```python
from build123d import *

# Parameters (mm, degrees)
F0_R            = 60
F1_DEPTH        = 6
F3_D            = 3.2
F6_D            = 3.2
F6_COPIES_COUNT = 5


# Not quite as in the source:
# - a pattern or mirror of a feature is missing from the dataset's text; its kind, count and spacing are read off the source's solid


with BuildPart() as f1:
    # F0 (on Top) → F1 (new body)
    with BuildSketch(Plane.XY):
        Circle(F0_R)
    extrude(amount=F1_DEPTH)

    # F3 (through all)
    with Locations(Plane.XY.offset(6)):
        with Locations((0, 0)):
            Hole(F3_D / 2)

    # F6 (through all)
    with Locations(Plane.XY.offset(6)):
        with Locations((0, 42.5)):
            f6 = Hole(F6_D / 2)

    # F6_copies: F6 ×5 about axis
    f6_copies_axis = Axis((0, 0, 0), (0, 0, 1))
    for i in range(1, F6_COPIES_COUNT):
        add(f6.rotate(f6_copies_axis, i * 360 / F6_COPIES_COUNT), mode=Mode.SUBTRACT)


solid = f1.part
```
Here's how the part is built. I have some questions about the finished solid (model axes, mm). Give positions to 0.01 mm unless a question says otherwise; leave off trailing zeros. Loops run counter-clockwise (first coordinate to the right, second up) from the corner with the lowest first, then second, coordinate; pieces in that order, holes last. Notation, with made-up numbers: M 76,-16 L 92,-16 A9 ccw 92,-7 Z; hole C 36,-24 d8. An arc over 180 degrees is marked long. Return JSON: item names as keys, results as strings.
Item 1: Imagine slicing it at B-B on x = 0. List the corners of the cut face in (y, z) for me.
A:
{"outline": "M -60,0 L -1.6,0 L -1.6,6 L -60,6 Z; M 1.6,0 L 40.9,0 L 40.9,6 L 1.6,6 Z; M 44.1,0 L 60,0 L 60,6 L 44.1,6 Z"}
Item 2: Please list where these lines run through material, in increasing order: line 1 (Y direction, x = 0, z = 3.6); line 2 (Y direction, x = -1, z = 2.2); line 3 (X direction, y = -33.5, z = 2.5) (3 decimals).
A:
{"line 1": "y = -60 to -1.6, 1.6 to 40.9, 44.1 to 60", "line 2": "y = -59.99 to -1.25, 1.25 to 41.25, 43.75 to 59.99", "line 3": "x = -49.777 to -26.315, -23.647 to 23.647, 26.315 to 49.777"}
Item 3: I'm going to push flat-ended pins straight in: pin 1 Ø2 at (x, z) = (-20, 2.5) entering from -Y; pin 2 Ø1 at (x, z) = (-47.5, 3.5) entering from -Y; pin 3 Ø1.5 at (x, z) = (46, 4.5) entering from -Y. Where does each tip first touch, or does it pass through?
A:
{"pin 1": "stops at y = -56.91", "pin 2": "stops at y = -37.3", "pin 3": "stops at y = -39.4"}
Item 4: Thinking about a two-plate mould opening in Y: for faces 1 (the cylindrical face through (-59.94, 2.64, 2.96)), 2 (the cylindrical face through (41.993, 13.425, 2.958)), 3 (the flat face through (12, 1, 0)), which applies, released by +Y, released by -Y, zero draft, split by the parting line, or undercut?
A:
{"face 1": "split by the parting line", "face 2": "undercut", "face 3": "zero draft"}
Item 5: Imagine slicing it at D-D on y = 42.5. List the corners of the cut face in (x, z) for me, then the cut area to 3 significant figures.
A:
{"outline": "M -42.35,0 L -1.6,0 L -1.6,6 L -42.35,6 Z; M 1.6,0 L 42.35,0 L 42.35,6 L 1.6,6 Z", "area": "489 mm^2"}
Item 6: Imagine slicing it at C-C on z = 2.65. List the corners of the cut face in (x, y) for me, then the cut area to 3 significant figures.
A:
{"outline": "C 0,0 d120; hole C -40.42,13.13 d3.2; hole C -24.98,-34.38 d3.2; hole C 0,0 d3.2; hole C 0,42.5 d3.2; hole C 24.98,-34.38 d3.2; hole C 40.42,13.13 d3.2", "area": "11,300 mm^2"}
Item 7: Imagine slicing it at A-A on y = 0. List the corners of the cut face in (x, z) for me.
A:
{"outline": "M -60,0 L -1.6,0 L -1.6,6 L -60,6 Z; M 1.6,0 L 60,0 L 60,6 L 1.6,6 Z"}
